Design review of the part built by this model. Coordinates are the model's own, in mm. A direction names the side the tool comes from. Coordinates: 2 decimals unless noted, no trailing zeros. Loops run counter-clockwise (first coordinate to the right, second up) from the corner with the lowest first, then second, coordinate; pieces in that order, holes last. Notation, with made-up numbers: (11.25, 71) - (46.25, 71) arc R10 ccw to (46.25, 85) - close; hole circle Ø1 at (76, 13). An arc over 180 degrees is marked (long way). One line per question, with ' | ' between items.
Autodesk Inventor part; units mm, degrees
ref_plane "YZ Plane" through (0, 0, 0) normal (1, 0, 0) x (0, 1, 0)
ref_plane "XZ Plane" through (0, 0, 0) normal (0, 1, 0) x (-1, 0, 0)
ref_plane "XY Plane" through (0, 0, 0) normal (0, 0, 1) x (1, 0, 0)
sketch "Sketch1" plane through (0, 0, 0) normal (0, 0, 1) x (1, 0, 0)
  line L0 (-12.7, 7.62) -> (12.7, 7.62) construction
  line L1 (-12.7, -7.62) -> (12.7, 7.62) construction
  line L2 (-12.7, 7.62) -> (12.7, -7.62) construction
  line L3 (-6.35, -11.7818) -> (-6.35, 0) construction
  line L4 (-2.54, 0) -> (2.54, 0)
  line L5 (6.35, 0) -> (6.35, -11.7818) construction
  line L6 (-6.35, -12.954) -> (6.35, 0) construction
  line L7 (-6.35, 0) -> (6.35, -12.954) construction
  line L8 (-25.5271, -12.954) -> (-6.35, -12.954) construction
  line L9 (0, -12.954) -> (34.2013, -12.954) construction
  line L10 (-6.35, -7.62) -> (-12.7, -7.62) construction
  line L11 (12.7, -7.62) -> (6.35, -7.62) construction
  line L12 (-12.7, 7.62) -> (-12.7, 12.7)
  line L13 (-12.7, 12.7) -> (12.7, 12.7) construction
  line L14 (12.7, 12.7) -> (12.7, 7.62)
  arc A0 (-12.7, -7.62) -> (-6.35, -11.7818) centre (0, 4.832) ccw construction
  arc A1 (6.35, -11.7818) -> (12.7, -7.62) centre (0, 4.832) ccw
  line L15 (-12.7, 2.667) -> (-16.51, 2.667) construction
  line L16 (-16.51, 4.953) -> (-12.7, 4.953) construction
  line L17 (-8.89, 4.953) -> (-8.89, 2.667) construction
  line L18 (-8.89, 2.667) -> (-16.51, 4.953) construction
  line L19 (-16.51, 2.667) -> (-8.89, 4.953) construction
  line L20 (12.7, 2.667) -> (16.51, 2.667) construction
  line L21 (16.51, 4.953) -> (12.7, 4.953) construction
  line L22 (8.89, 4.953) -> (8.89, 2.667) construction
  line L23 (8.89, 2.667) -> (16.51, 4.953) construction
  line L24 (16.51, 2.667) -> (8.89, 4.953) construction
  line L25 (-12.7, -7.62) -> (-12.7, 2.286)
  line L26 (12.7, 2.286) -> (12.7, -7.62)
  line L27 (-12.7, 12.7) -> (12.7, 12.7)
  line L28 (-16.51, 4.953) -> (-16.51, 5.334)
  line L29 (6.35, 0) -> (5.715, 0) construction
  line L30 (-6.35, 0) -> (-5.715, 0) construction
  line L31 (-5.715, 0) -> (-5.715, -0.6477) construction
  line L32 (5.715, 0) -> (5.715, -0.6477) construction
  arc A2 (-6.35, -11.7818) -> (-5.715, -12.0108) centre (0, 4.832) ccw
  arc A3 (5.715, -12.0108) -> (6.35, -11.7818) centre (0, 4.832) ccw
  line L33 (-12.7, -7.62) -> (12.7, -7.62) construction
  line L34 (-5.715, 0) -> (-3.175, 0) construction
  line L35 (5.715, 0) -> (3.175, 0) construction
  arc A4 (-6.35, -11.7818) -> (-5.4965, -12.0834) centre (0, 4.832) ccw
  arc A5 (3.175, -12.6683) -> (12.7, -7.62) centre (0, 4.832) ccw
  line L36 (-12.7, 7.62) -> (-16.51, 7.62)
  line L37 (-16.51, 7.62) -> (-16.51, 4.572)
  line L38 (-16.51, 4.572) -> (-12.7, 4.572)
  line L39 (-12.7, 4.572) -> (-12.7, 1.9405)
  line L40 (12.7, 7.62) -> (16.51, 7.62)
  line L41 (16.51, 7.62) -> (16.51, 4.572)
  line L42 (16.51, 4.572) -> (12.7, 4.572)
  line L43 (12.7, 4.572) -> (12.7, 2.286)
  line L44 (-3.175, 0) -> (-2.54, 0) construction
  line L45 (-2.54, 0) -> (-2.54, -12.7717)
  line L46 (3.175, 0) -> (2.54, 0) construction
  line L47 (2.54, 0) -> (2.54, -12.7717)
  arc A6 (-12.7, -7.62) -> (-2.54, -12.7717) centre (0, 4.832) ccw
  arc A7 (2.54, -12.7717) -> (12.7, -7.62) centre (0, 4.832) ccw
  point P0 (0, 0)
  point P1 (0, -6.477)
  point P2 (-12.7, 3.81)
  point P3 (12.7, 3.81)
  dimension "d0" = 15.24
  dimension "d1" = 25.4
  dimension "d3" = 12.7
  dimension "d4" = 5.08
  dimension "d5" = 1.1722
  dimension "d7" = 7.62
  dimension "d8" = 2.286
  dimension "d9" = 7.62
  dimension "d17" = 0.635
  dimension "d18" = 0.635
  dimension "d19" = 90
  dimension "d22" = 2.54
  dimension "d24" = 2.54
  dimension "d30" = 3.81
  dimension "d31" = 3.048
  dimension "d33" = 3.81
  dimension "d36" = 0.635
  dimension "d37" = 0.635
extrude "Extrusion6" add sketch "Sketch1" along normal mid plane 5.08
sketch "Sketch2" plane through (0, 0, 2.54) normal (0, 0, 1) x (1, 0, 0)
  line L0 (-12.7, 4.572) -> (-12.7, -7.62)
  arc A0 (-12.7, -7.62) -> (-2.54, -12.7717) centre (0, 4.832) ccw
  line L1 (-2.54, -12.7717) -> (-2.54, 0)
  line L2 (-2.54, 0) -> (2.54, 0)
  line L3 (2.54, 0) -> (2.54, -12.7717)
  arc A1 (2.54, -12.7717) -> (12.7, -7.62) centre (0, 4.832) ccw
  line L4 (12.7, -7.62) -> (12.7, 4.572)
  line L5 (12.7, 4.572) -> (16.51, 4.572)
  line L6 (16.51, 4.572) -> (16.51, 7.62)
  line L7 (16.51, 7.62) -> (12.7, 7.62)
  line L8 (12.7, 7.62) -> (12.7, 12.7)
  line L9 (12.7, 12.7) -> (-12.7, 12.7)
  line L10 (-12.7, 12.7) -> (-12.7, 7.62)
  line L11 (-12.7, 7.62) -> (-16.51, 7.62)
  line L12 (-16.51, 7.62) -> (-16.51, 4.572)
  line L13 (-16.51, 4.572) -> (-12.7, 4.572)
  point P0 (0, 0)
properties part number "BottomPegCor"
Q1. Take a section at D-D (y = -8.5). Give the boundary of the cut face in (x, z), plus the area to 3 significant figures.
Returned:
outline: (-11.77, -2.54) - (-2.54, -2.54) - (-2.54, 2.54) - (-11.77, 2.54) - close; (2.54, -2.54) - (11.77, -2.54) - (11.77, 2.54) - (2.54, 2.54) - close | area: 93.8 mm²
Q2. Take a section at C-C (x = -1). Give the boundary of the cut face in (y, z).
Returned:
outline: (0, -2.54) - (12.7, -2.54) - (12.7, 2.54) - (0, 2.54) - close
Q3. For pin 1 (1.5 mm diameter, centred on y = -7.5, z = -0.5, fed in from +X); pin 2 (1.1 mm diameter, centred on x = 15.5, z = 1, fed in from +Y); pin 3 (1.5 mm diameter, centred on x = 7, z = 1.5, fed in from -Y), all flat-tipped, find the tip position at first contact; note any pin that passes through.
Returned:
pin 1: stops at x = 12.7 | pin 2: stops at y = 7.62 | pin 3: stops at y = -11.82
Q4. To check wall thickness, follow line 1 along X through (y, z) = (-1.75, -1); line 2 along Y through (x, z) = (2, 1.75); line 3 along X through (y, z) = (-10.75, -0.95). State the ranges of each line that lie inside material, in increasing order.
Returned:
line 1: x = -12.7 to -2.54, 2.54 to 12.7 | line 2: y = 0 to 12.7 | line 3: x = -8.58 to -2.54, 2.54 to 8.58
Q5. Take a section at A-A (y = -1). Give the boundary of the cut face in (x, z), plus the area to 3 significant figures.
Returned:
outline: (-12.7, -2.54) - (-2.54, -2.54) - (-2.54, 2.54) - (-12.7, 2.54) - close; (2.54, -2.54) - (12.7, -2.54) - (12.7, 2.54) - (2.54, 2.54) - close | area: 103 mm²
Q6. Tool access review of faces 1 (the flat face through (-12.7, 10, 0)), 2 (the flat face through (12.7, 10, 0)), 3 (the flat face through (0, 0, 0)), 4 (the flat face through (-15, 4.572, 0)), 5 (the flat face through (12.7, -1, 0)): name each direction out of +Z, -Z, +X, -X, +Y, -Y from which nothing blocks a thin tool from reaching the whole face with its end or side.
Returned:
face 1: +Z, -Z, -X, +Y | face 2: +Z, -Z, +X, +Y | face 3: +Z, -Z, -Y | face 4: +Z, -Z, -X, -Y | face 5: +Z, -Z, +X, -Y
Q7. Draft analysis for pull direction X (two halves, no side actions). For faces 6 (the flat face through (16.51, 6, 0)), 7 (the flat face through (2.54, -6, 0)), 8 (the flat face through (15, 7.62, 0)), state which applies: +X half, -X half, draft (parallel to the pull), parting line (faces both ways), or undercut.
Returned:
face 6: +X half | face 7: undercut | face 8: draft
